```python
from build123d import *

# Parameters (mm, degrees)
F0_W     = 140
F0_H     = 75
F1_DEPTH = 5
F2_W     = 12.5
F2_H     = 12.5
F3_DEPTH = 25
F4_R     = 12.5
F5_DEPTH = 25
F7_DEPTH = 25


with BuildPart() as f1:
    # F0 (on Top) → F1 (new body)
    with BuildSketch(Plane.XY):
        with Locations((2.230102, 8.409632)):
            Rectangle(F0_W, F0_H)
    extrude(amount=F1_DEPTH)

    # F2 (on face) → F3 (cut)
    with BuildSketch(Plane.XY.offset(5)):
        with Locations((-56.519898, 35.497632)):
            Rectangle(F2_W, F2_H)
        with Locations((60.980102, 35.497632)):
            Rectangle(F2_W, F2_H)
    extrude(amount=-F3_DEPTH, mode=Mode.SUBTRACT)

    # F4 (on face) → F5 (cut)
    with BuildSketch(Plane.XY.offset(5)):
        with Locations((2.230102, -4.090368)):
            Circle(F4_R)
    extrude(amount=-F5_DEPTH, mode=Mode.SUBTRACT)

    # F6 (on face) → F7 (cut)
    with BuildSketch(Plane.XY.offset(5)):
        Polygon((-32.769898, -29.090368), (-67.769898, 8.409632), (-67.769898, -29.090368), align=None)
        Polygon((72.230102, -29.090368), (72.230102, 8.409632), (37.230102, -29.090368), align=None)
    extrude(amount=-F7_DEPTH, mode=Mode.SUBTRACT)


solid = f1.part
```
Can you work these out from the model? Positions are in its coordinate system, mm. A direction names the side the tool comes from. Coordinates: 2 decimals unless noted, no trailing zeros. Write each loop counter-clockwise with the first axis right and the second up, starting at its lowest first coordinate (ties: lowest second). Pieces come first, ordered by that corner, then holes. Notation, with made-up numbers: (79, 52) - (101, 52) arc R23 cw to (101, 77) - close; hole circle Ø8 at (42, 12). An arc over 180 degrees is marked (long way). Return JSON: item names as keys, results as strings.
Q1. If we section it at C-C (z = 3.4): Please give me the cut outline in (x, y).
Computed values:
{"outline": "(-67.77, 8.41) - (-32.77, -29.09) - (37.23, -29.09) - (72.23, 8.41) - (72.23, 45.91) - (-67.77, 45.91) - close; hole (-62.77, 29.25) - (-50.27, 29.25) - (-50.27, 41.75) - (-62.77, 41.75) - close; hole circle Ø25 at (2.23, -4.09); hole (54.73, 29.25) - (67.23, 29.25) - (67.23, 41.75) - (54.73, 41.75) - close"}
Q2. If we section it at A-A (y = 36): Please give me the cut outline in (x, z), then the cut area to 3 significant figures.
Computed values:
{"outline": "(-67.77, 0) - (-62.77, 0) - (-62.77, 5) - (-67.77, 5) - close; (-50.27, 0) - (54.73, 0) - (54.73, 5) - (-50.27, 5) - close; (67.23, 0) - (72.23, 0) - (72.23, 5) - (67.23, 5) - close", "area": "575 mm2"}
Q3. If we section it at D-D (y = -2): Please give me the cut outline in (x, z).
Computed values:
{"outline": "(-58.05, 0) - (-10.09, 0) - (-10.09, 5) - (-58.05, 5) - close; (14.55, 0) - (62.51, 0) - (62.51, 5) - (14.55, 5) - close"}
Q4. Please list where these lines run through material, in increasing order: L1, parallel to X at y = 38.5, z = 2.4; L2, parallel to Y at x = 62, z = 3.85; L3, parallel to X at y = -2.5, z = 4.35. Write a range as from..to.
Computed values:
{"L1": "x = -67.77..-62.77, -50.27..54.73, 67.23..72.23", "L2": "y = -2.55..29.25, 41.75..45.91", "L3": "x = -57.59..-10.17, 14.63..62.05"}
Q5. I'm going to push a flat-ended pin straight in: pin 1 Ø2.5 at (x, z) = (-58, 1.5) entering from -Y. Where does the tip first touch, or does it pass through?
Computed values:
{"pin 1": "stops at y = -3.4"}
Q6. On a 3-axis mill with a long thin cutter (end or side, diameter ignored), from which of +Z, -Z, +X, -X, +Y, -Y can I reach the whole of each face in a straight line? I mean faces 5 (the flat face through (-67.77, 27, 2)), 6 (the flat face through (-57, 41.748, 3)). Say none if no direction works.
Computed values:
{"face 5": "+Z, -Z, -X, +Y, -Y", "face 6": "+Z, -Z"}
Q7. If we section it at B-B (x = -55): Please give me the cut outline in (y, z).
Computed values:
{"outline": "(-5.27, 0) - (29.25, 0) - (29.25, 5) - (-5.27, 5) - close; (41.75, 0) - (45.91, 0) - (45.91, 5) - (41.75, 5) - close"}
Q8. Thinking about a two-plate mould opening in Y: for faces 1 (the flat face through (1, 9, 5)), 2 (the cylindrical face through (-7.689, -11.696, 2.535)), 3 (the flat face through (-50.27, 35, 3)), 4 (the flat face through (2, -29.09, 2)), which applies, +Y half, -Y half, draft (parallel to the pull), parting line (faces both ways), or undercut?
Computed values:
{"face 1": "draft", "face 2": "undercut", "face 3": "undercut", "face 4": "-Y half"}
